Here's how the part is built. I have some questions about the finished solid (model axes, mm). Face numbers are marked on the shaded views. A direction names the side the tool comes from. Round coordinates to 2 decimals unless told otherwise and drop trailing zeros. Write each loop counter-clockwise with the first axis right and the second up, starting at its lowest first coordinate (ties: lowest second). Pieces come first, ordered by that corner, then holes. Notation, with made-up numbers: (10, 89.25) - (32, 89.25) arc R21 cw to (32, 110.25) - close; hole circle Ø1 at (-37, 6.25). An arc over 180 degrees is marked (long way). One line per question, with ' | ' between items. Start each with the question number.
(1) Will these pins go through, and if not, where does the flat tip stop? pin 1 (5 mm diameter, centred on x = 21.5, y = -20, fed in from -Z); pin 2 (3.5 mm diameter, centred on y = -77.5, z = 7, fed in from +X); pin 3 (6 mm diameter, centred on y = -13, z = 16, fed in from +X); pin 4 (14.5 mm diameter, centred on y = -7, z = 13, fed in from +X).
(2) If I drill on L1, parallel to X at y = 26, z = 8.5; L2, parallel to Y at x = 10, z = 23.5; L3, parallel to Y at x = -23, z = 21.75, over which ranges is the centre line in solid material (lowest first)?
(3) Imagine slicing it at A-A (y = -11). Write out the boundary of the cut face in (x, z).
(4) Imagine slicing it at C-C (z = 9.5). Write out the boundary of the cut face in (x, y) (3 decimals), plus the area to 3 significant figures.
(5) Imagine slicing it at D-D (x = -9). Write out the boundary of the cut face in (y, z).
(6) Imagine slicing it at B-B (x = 28.5). Write out the boundary of the cut face in (y, z).
(7) Thinking about a two-plate mould opening in X: for the marked faces 5, 6, 7 and 8, which applies, pulls with the +X half, pulls with the -X half, needs draft (parallel to the pull), parting line crosses it, or undercut?
(8) For the marked faces 1, 2, 3 and 4, which set-ups out of +Z, -Z, +X, -X, +Y, -Y let a thin tool reach every point of the face, with its end or its side?
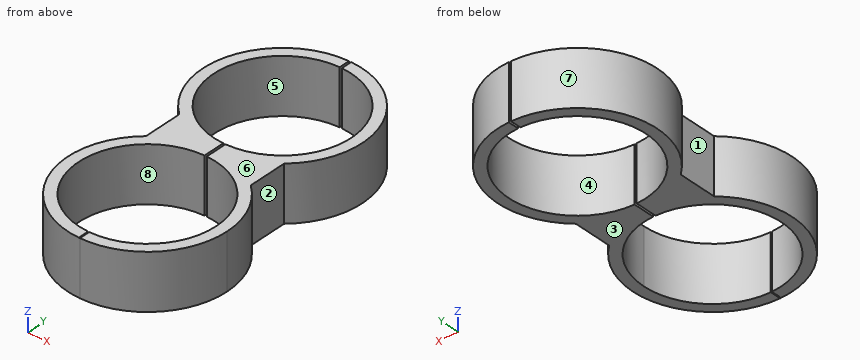
from build123d import *

# Parameters (mm, degrees)
F1_DEPTH = 25


with BuildPart() as f1:
    # F0 (on Top) → F1 (new body)
    with BuildSketch(Plane.XY):
        with BuildLine():
            ThreePointArc((-0.5, -3.905880259), (-31.125, 27.2151034176), (-0.5, 58.3360870942))
            Line((-0.5, 58.3360870942), (-0.5, 63.3366430443))
            ThreePointArc((-0.5, 63.3366430443), (-33.9112453853, 39.6667322838), (-23.756131229, 0))
            ThreePointArc((-23.756131229, 0), (-12.9197959363, -6.5205527634), (-0.5, -8.906436209))
            Line((-0.5, -8.906436209), (-0.5, -3.905880259))
        make_face()
        with BuildLine():
            Line((-0.5, -8.9133569557), (-0.5, -8.906436209))
            ThreePointArc((-0.5, -8.906436209), (-12.9197959363, -6.5205527634), (-23.756131229, 0))
            Line((-23.756131229, 0), (-23.756131229, -17.8197931647))
            ThreePointArc((-23.756131229, -17.8197931647), (-12.9197959363, -11.2992404013), (-0.5, -8.9133569557))
        make_face()
        with BuildLine():
            ThreePointArc((0.5, 58.3360870942), (31.125, 27.2151034176), (0.5, -3.905880259))
            Line((0.5, -3.905880259), (0.5, -8.906436209))
            ThreePointArc((0.5, -8.906436209), (12.9197959363, -6.5205527634), (23.756131229, 0))
            ThreePointArc((23.756131229, 0), (33.9112453853, 39.6667322838), (0.5, 63.3366430443))
            Line((0.5, 63.3366430443), (0.5, 58.3360870942))
        make_face()
        with BuildLine():
            Line((-0.5, -13.9139129058), (-0.5, -8.9133569557))
            ThreePointArc((-0.5, -8.9133569557), (-12.9197959363, -11.2992404013), (-23.756131229, -17.8197931647))
            ThreePointArc((-23.756131229, -17.8197931647), (-33.8242607899, -57.7209127821), (0, -81.1598965824))
            Line((0, -81.1598965824), (0, -80.5474147201))
            Line((0, -80.5474147201), (-0.5, -80.5474147201))
            Line((-0.5, -80.5474147201), (-0.5, -76.155880259))
            ThreePointArc((-0.5, -76.155880259), (-31.125, -45.0348965824), (-0.5, -13.9139129058))
        make_face()
        with BuildLine():
            ThreePointArc((23.756131229, 0), (12.9197959363, -6.5205527634), (0.5, -8.906436209))
            Line((0.5, -8.906436209), (0.5, -8.9133569557))
            ThreePointArc((0.5, -8.9133569557), (12.9197959363, -11.2992404013), (23.756131229, -17.8197931647))
            Line((23.756131229, -17.8197931647), (23.756131229, 0))
        make_face()
        with BuildLine():
            ThreePointArc((23.756131229, -17.8197931647), (12.9197959363, -11.2992404013), (0.5, -8.9133569557))
            Line((0.5, -8.9133569557), (0.5, -13.9139129058))
            ThreePointArc((0.5, -13.9139129058), (22.1847709589, -23.2036904201), (31.125, -45.0348965824))
            ThreePointArc((31.125, -45.0348965824), (22.1847709589, -66.8661027446), (0.5, -76.155880259))
            ThreePointArc((0.5, -76.155880259), (0.2500080653, -76.1588924853), (0, -76.1598965824))
            Line((0, -76.1598965824), (0, -80.5474147201))
            Line((0, -80.5474147201), (0, -81.1598965824))
            ThreePointArc((0, -81.1598965824), (25.5442324704, -70.5791290527), (36.125, -45.0348965824))
            ThreePointArc((36.125, -45.0348965824), (32.8877322542, -30.0879004903), (23.756131229, -17.8197931647))
        make_face()
    extrude(amount=F1_DEPTH)


solid = f1.part
Check sheet entries:
1) pin 1: z = 0 | pin 2: x = 19.02 | pin 3: x = 23.76 | pin 4: x = 24.04
2) L1: -36.1 to -31.1, 31.1 to 36.1 | L2: -79.75 to -74.51, -15.56 to -2.26, 56.69 to 61.93 | L3: -72.89 to -66.01, -24.06 to 6.24, 48.19 to 55.07
3) outline: (-23.76, 0) - (-0.5, 0) - (-0.5, 25) - (-23.76, 25) - close; (0.5, 0) - (23.76, 0) - (23.76, 25) - (0.5, 25) - close
4) outline: (-23.756, -17.82) arc R36.125 ccw (long way) to (23.756, -17.82) - (23.756, 0) arc R36.125 ccw to (0.5, 63.337) - (0.5, 58.336) arc R31.125 cw to (0.5, -3.906) - (0.5, -13.914) arc R31.125 cw to (0.5, -76.156) arc R31.125 cw to (0, -76.16) - (0, -80.547) - (-0.5, -80.547) - (-0.5, -76.156) arc R31.125 cw to (-0.5, -13.914) - (-0.5, -3.906) arc R31.125 cw to (-0.5, 58.336) - (-0.5, 63.337) arc R36.125 ccw to (-23.756, 0) - close | area: 2,360 mm^2
5) outline: (-80.02, 0) - (-74.83, 0) - (-74.83, 25) - (-80.02, 25) - close; (-15.24, 0) - (-2.58, 0) - (-2.58, 25) - (-15.24, 25) - close; (57.01, 0) - (62.2, 0) - (62.2, 25) - (57.01, 25) - close
6) outline: (-67.23, 0) - (-57.55, 0) - (-57.55, 25) - (-67.23, 25) - close; (-32.52, 0) - (-22.84, 0) - (-22.84, 25) - (-32.52, 25) - close; (5.02, 0) - (14.7, 0) - (14.7, 25) - (5.02, 25) - close; (39.73, 0) - (49.41, 0) - (49.41, 25) - (39.73, 25) - close
7) face 5: undercut | face 6: needs draft | face 7: pulls with the -X half | face 8: undercut
8) face 1: +Z, -Z, -X | face 2: +Z, -Z, +X | face 3: -Z, +X, -X, +Y, -Y | face 4: +Z, -Z
